Source: CAD feature listing. Evaluate the final solid. Frame: model axes, mm. A direction names the side the tool comes from. Coordinates: 2 decimals unless noted, no trailing zeros. Loops run counter-clockwise (first coordinate to the right, second up) from the corner with the lowest first, then second, coordinate; pieces in that order, holes last. Notation, with made-up numbers: M 53,45 L 95,45 A14 cw 95,50 Z; hole C -27.5,-3 d2. An arc over 180 degrees is marked long. Write each question's results on one line, items separated by ' | '. Start each with the question number.
from build123d import *

# Parameters (mm, degrees)
SKETCH1_W                   = 80
SKETCH1_H                   = 40
BOSS_EXTRUDE1_DEPTH         = 12
FILLET1_RADIUS              = 20
FILLET1_LENGTH              = 12
SKETCH2_W                   = 50
SKETCH2_H                   = 15
BOSS_EXTRUDE2_DEPTH         = 40
FILLET3_RADIUS              = 25
FILLET3_LENGTH              = 15
SKETCH4_R                   = 8
CUT_EXTRUDE2_DEPTH          = 40
FILLET3_OF_MIRROR7_2_RADIUS = 25
FILLET3_OF_MIRROR7_2_LENGTH = 15
SKETCH5_R                   = 8
CUT_EXTRUDE4_DEPTH          = 40
SKETCH7_W                   = 12
SKETCH7_H                   = 40
BOSS_EXTRUDE3_DEPTH         = 40
FILLET4_RADIUS              = 20
FILLET4_LENGTH              = 12
SKETCH8_R                   = 8
CUT_EXTRUDE5_DEPTH          = 40
FILLET6_R                   = 2
FILLET7_R                   = 2
FILLET8_R                   = 2
FILLET9_R                   = 2
FILLET10_R                  = 2


with BuildPart() as part:
    # Sketch1 → Boss-Extrude1 (new body)
    with BuildSketch(Plane(origin=(0, 0, 0), x_dir=(1, 0, 0), z_dir=(0, 1, 0))):
        Rectangle(SKETCH1_W, SKETCH1_H)
    extrude(amount=BOSS_EXTRUDE1_DEPTH)

    # Fillet1: full round fillet: the end face becomes a half cylinder, R = half its width
    fillet1_face = Plane((40, 6, 0), x_dir=(0, -1, 0), z_dir=(1, 0, 0))  # on the end face: x along it, z out of the body
    fillet1_slab = fillet1_face.offset(-FILLET1_RADIUS / 2) * Box(FILLET1_LENGTH, 2 * FILLET1_RADIUS, FILLET1_RADIUS, mode=Mode.PRIVATE)  # the body's end, R deep
    fillet1_round = Plane((20, 6, 0), x_dir=(1, 0, 0), z_dir=(0, -1, 0)) * Cylinder(FILLET1_RADIUS, FILLET1_LENGTH, mode=Mode.PRIVATE)  # its axis R under the face
    add(fillet1_slab - fillet1_round, mode=Mode.SUBTRACT)

    # Sketch2 → Boss-Extrude2 (add)
    with BuildSketch(Plane(origin=(0, 12, 0), x_dir=(1, 0, 0), z_dir=(0, 1, 0))):
        with Locations((-15, -12.5)):
            Rectangle(SKETCH2_W, SKETCH2_H)
    boss_extrude2 = extrude(amount=BOSS_EXTRUDE2_DEPTH)

    # Fillet3: full round fillet: the end face becomes a half cylinder, R = half its width
    fillet3_face = Plane((-15, 52, 12.5), x_dir=(0, 0, 1), z_dir=(0, 1, 0))  # on the end face: x along it, z out of the body
    fillet3_slab = fillet3_face.offset(-FILLET3_RADIUS / 2) * Box(FILLET3_LENGTH, 2 * FILLET3_RADIUS, FILLET3_RADIUS, mode=Mode.PRIVATE)  # the body's end, R deep
    fillet3_round = Plane((-15, 27, 12.5), x_dir=(0, 1, 0), z_dir=(0, 0, 1)) * Cylinder(FILLET3_RADIUS, FILLET3_LENGTH, mode=Mode.PRIVATE)  # its axis R under the face
    add(fillet3_slab - fillet3_round, mode=Mode.SUBTRACT)

    # Sketch4 → Cut-Extrude2 (cut)
    with BuildSketch(Plane.XY.offset(20)):
        with Locations((-15, 27)):
            Circle(SKETCH4_R)
    cut_extrude2 = extrude(amount=-CUT_EXTRUDE2_DEPTH, mode=Mode.SUBTRACT)

    # Mirror7: Boss-Extrude2, Cut-Extrude2 across plane
    add(boss_extrude2.mirror(Plane.XY))
    add(cut_extrude2.mirror(Plane.XY), mode=Mode.SUBTRACT)

    # Fillet3 of Mirror7 2: full round fillet: the end face becomes a half cylinder, R = half its width
    fillet3_of_mirror7_2_face = Plane((-15, 52, -12.5), x_dir=(0, 0, -1), z_dir=(0, 1, 0))  # on the end face: x along it, z out of the body
    fillet3_of_mirror7_2_slab = fillet3_of_mirror7_2_face.offset(-FILLET3_OF_MIRROR7_2_RADIUS / 2) * Box(FILLET3_OF_MIRROR7_2_LENGTH, 2 * FILLET3_OF_MIRROR7_2_RADIUS, FILLET3_OF_MIRROR7_2_RADIUS, mode=Mode.PRIVATE)  # the body's end, R deep
    fillet3_of_mirror7_2_round = Plane((-15, 27, -12.5), x_dir=(0, 1, 0), z_dir=(0, 0, -1)) * Cylinder(FILLET3_OF_MIRROR7_2_RADIUS, FILLET3_OF_MIRROR7_2_LENGTH, mode=Mode.PRIVATE)  # its axis R under the face
    add(fillet3_of_mirror7_2_slab - fillet3_of_mirror7_2_round, mode=Mode.SUBTRACT)

    # Sketch5 → Cut-Extrude4 (cut)
    with BuildSketch(Plane(origin=(0, 12, 0), x_dir=(1, 0, 0), z_dir=(0, 1, 0))):
        with Locations(Location((20, 0, 0), (0, 0, 270))):
            Circle(SKETCH5_R)
    extrude(amount=-CUT_EXTRUDE4_DEPTH, mode=Mode.SUBTRACT)

    # Sketch7 → Boss-Extrude3 (add)
    with BuildSketch(Plane(origin=(0, 0, 0), x_dir=(-1, 0, 0), z_dir=(0, -1, 0))):
        with Locations((34, 0)):
            Rectangle(SKETCH7_W, SKETCH7_H)
    extrude(amount=BOSS_EXTRUDE3_DEPTH)

    # Fillet4: full round fillet: the end face becomes a half cylinder, R = half its width
    fillet4_face = Plane((-34, -40, 0), x_dir=(1, 0, 0), z_dir=(0, -1, 0))  # on the end face: x along it, z out of the body
    fillet4_slab = fillet4_face.offset(-FILLET4_RADIUS / 2) * Box(FILLET4_LENGTH, 2 * FILLET4_RADIUS, FILLET4_RADIUS, mode=Mode.PRIVATE)  # the body's end, R deep
    fillet4_round = Plane((-34, -20, 0), x_dir=(0, -1, 0), z_dir=(1, 0, 0)) * Cylinder(FILLET4_RADIUS, FILLET4_LENGTH, mode=Mode.PRIVATE)  # its axis R under the face
    add(fillet4_slab - fillet4_round, mode=Mode.SUBTRACT)

    # Sketch8 → Cut-Extrude5 (cut)
    with BuildSketch(Plane.ZY.offset(40)):
        with Locations((0, -20)):
            Circle(SKETCH8_R)
    extrude(amount=-CUT_EXTRUDE5_DEPTH, mode=Mode.SUBTRACT)

    # Fillet6
    fillet6_edges = [part.edges().sort_by_distance(p)[0] for p in [
        (10, 12, 12.5),
    ]]
    fillet(fillet6_edges, radius=FILLET6_R)

    # Fillet7
    fillet7_edges = [part.edges().sort_by_distance(p)[0] for p in [
        (-14, 12, 5),
    ]]
    fillet(fillet7_edges, radius=FILLET7_R)

    # Fillet8
    fillet8_edges = [part.edges().sort_by_distance(p)[0] for p in [
        (-15, 12, -5),
    ]]
    fillet(fillet8_edges, radius=FILLET8_R)

    # Fillet9
    fillet9_edges = [part.edges().sort_by_distance(p)[0] for p in [
        (10, 12, -11.5),
    ]]
    fillet(fillet9_edges, radius=FILLET9_R)

    # Fillet10
    fillet10_edges = [part.edges().sort_by_distance(p)[0] for p in [
        (-28, 0, 0),
    ]]
    fillet(fillet10_edges, radius=FILLET10_R)


solid = part.part
Item 1: Cut plane A-A (z = 0). Output: boundary loops of the cut face in (x, y).
Item 2: Access query for faces 4 (the flat face through (10, 20, 13)), 5 (the cylindrical face through (-13.64, 12.6, 4.43)), 6 (the flat face through (7, 0, 0)). Directions: +Z, -Z, +X, -X, +Y, -Y. A direction counts if a zero-diameter tool reaches every point of the face in a straight line with its end or side. Return the directions, or none.
Item 3: Cut plane C-C (z = -12). Output: boundary loops of the cut face in (x, y).
Item 4: Cut plane B-B (x = -15). Output: boundary loops of the cut face in (y, z), then the cut area to 3 significant figures.
Item 5: Cut plane D-D (y = 29). Output: boundary loops of the cut face in (x, z), then the cut area to 3 significant figures.
Item 6: First-contact query: pin 1 Ø8 at (x, z) = (9, 11.5) entering from -Y; pin 2 Ø14.5 at (x, y) = (-15, 27) entering from -Z; pin 3 Ø8 at (x, z) = (-25, 13.5) entering from +Y; pin 4 Ø14.5 at (y, z) = (20.5, 14.5) entering from +X. Flat tips, straight axial feed; report the tip coordinate or a pass-through.
Item 7: Mould query, pull axis Z, two halves, no side actions, for faces 1 (the flat face through (-16, 17, 20)), 2 (the cylindrical face through (10.6, 12.57, 11.38)), 3 (the cylindrical face through (-34.08, -27.81, -1.73)). Classes: +Z half, -Z half, draft (parallel to the pull), parting line (faces both ways), or undercut.
Item 8: Line query: probe 1 along X at (y, z) = (27, -13.75); probe 2 along X at (y, z) = (2.5, 0); probe 3 along X at (y, z) = (-30.5, -3.5). Output: solid intervals per line, ascending.
Response values:
1) outline: M -40,-40 L -28,-40 L -28,-28 L -40,-28 Z; M -40,-12 L -28,-12 L -28,-2 A2 cw -26,0 L 12,0 L 12,12 L -40,12 Z; M 28,0 L 40,0 L 40,12 L 28,12 Z
2) face 4: +Z, -Z, +X, +Y | face 5: +X, -X, +Y | face 6: +Z, -Z, +X, -Y
3) outline: M -40,-36 L -28,-36 L -28,-2 A2 cw -26,0 L 36,0 L 36,12 L 12,12 A2 cw 10,14 L 10,27 A25 ccw -40,27 Z; hole C -15,27 d16
4) outline: M 0,-20 L 19,-20 L 19,-5 L 14,-5 A2 cw 12,-3 L 12,3 A2 cw 14,5 L 19,5 L 19,20 L 0,20 Z; M 35,-20 L 52,-20 L 52,-5 L 35,-5 Z; M 35,5 L 52,5 L 52,20 L 35,20 Z | area: 1,200 mm2
5) outline: M -39.92,-20 L -22.75,-20 L -22.75,-5 L -39.92,-5 Z; M -39.92,5 L -22.75,5 L -22.75,20 L -39.92,20 Z; M -7.25,-20 L 9.92,-20 L 9.92,-5 L -7.25,-5 Z; M -7.25,5 L 9.92,5 L 9.92,20 L -7.25,20 Z | area: 1,030 mm2
6) pin 1: stops at y = 0 | pin 2: passes through | pin 3: stops at y = 51.27 | pin 4: stops at x = 10.15
7) face 1: +Z half | face 2: draft | face 3: undercut
8) probe 1: x = -40 to -23, -7 to 10 | probe 2: x = -40 to 12, 28 to 40 | probe 3: x = -40 to -28
